The model under review builds one solid part; all positions refer to its coordinate system, in mm. A direction names the side the tool comes from. Coordinates: 2 decimals unless noted, no trailing zeros. Order: outer loops, then holes, each group sorted by start corner. A loop starts at its lowest first (then second) coordinate and runs counter-clockwise, first axis right, second up. Notation, with made-up numbers: (-9, 2.25) -> (10, 2.25) arc R18 ccw to (10, 30.25) -> close; hole circle Ø4 at (56.5, -20). An arc over 180 degrees is marked (long way). Use one line per item in the form item = value. Start each with the question number.
(1) Take a section at C-C (y = -6.5). State the section outline as (x, z) points, then the cut area to 3 significant figures.
(2) Wall thickness on line 1 along Y through (x, z) = (-6.75, 0.35); line 2 along Z through (x, y) = (-9.5, 4.5); line 3 along Y through (x, z) = (8, 0.9): over which ranges is each line inside the solid? List them lowest first.
(3) Take a section at A-A (y = 0.25). State the section outline as (x, z) points.
(4) Insertion check: pin 1 Ø0.5 at (x, z) = (7, 0.5) entering from +Y; pin 2 Ø0.7 at (y, z) = (-8, 2) entering from +X; pin 3 Ø1 at (x, z) = (8, 1.5) entering from -Y. Each pin has a flat end and moves straight along its axis. Give the tip position at first contact, or say it passes through.
(5) Mouldability with a two-part tool opening along X and no side actions: class faces 1 (the flat face through (-8, 9.45, 2)), 2 (the flat face through (-5.55, 7, 2)), 3 (the flat face through (-9.45, -7, 2)), 4 (the cylindrical face through (-5.72, -7.48, 1.09)) as +X half, -X half, draft (parallel to the pull), parting line (faces both ways), or undercut.
(6) Take a section at D-D (x = -7.25). State the section outline as (y, z) points.
(7) For faces 5 (the cylindrical face through (-7.527, -5.723, 1.082)), 6 (the flat face through (9.45, -7, 2)), 7 (the flat face through (-5.55, -7, 2)), 8 (the cylindrical face through (7.47, 9.28, 1.09)), list the 3-axis set-ups (+Z, -Z, +X, -X, +Y, -Y) from which the entire face can be reached by the end or side of a thin tool; tool diameter is ignored.
```python
from build123d import *

# Parameters (mm, degrees)
SKETCH_1_W          = 30
SKETCH_1_H          = 30
EXTRUDE_1_DEPTH     = 2
SKETCH_2_W          = 3
SKETCH_2_H          = 3
EXTRUDE_2_DEPTH     = 1
EXTRUDE_START       = 5
EXTRUDE_3_DEPTH     = 5
CUT_EXTRUDE_1_DEPTH = 29.793271784
FILLET_1_R          = 0.1
FILLET_2_R          = 0.2


with BuildPart() as part:
    # 草图1 → 凸台-拉伸1 (new body)
    with BuildSketch(Plane.XY):
        Rectangle(SKETCH_1_W, SKETCH_1_H)
    extrude(amount=-EXTRUDE_1_DEPTH)

    # 草图2 → 凸台-拉伸2 (add)
    with BuildSketch(Plane.XY):
        with Locations((-7.5, -7.5)):
            Rectangle(SKETCH_2_W, SKETCH_2_H)
        with Locations((7.5, -7.5)):
            Rectangle(SKETCH_2_W, SKETCH_2_H)
    extrude_2 = extrude(amount=EXTRUDE_2_DEPTH)

    # 草图3 → 凸台-拉伸3 (add)
    with BuildSketch(Plane.XZ.offset(EXTRUDE_START)):
        with BuildLine():
            Line((-9.45, 2.5), (-5.55, 2.5))
            Line((-5.55, 2.5), (-5.55, 1.555590279))
            ThreePointArc((-5.55, 1.555590279), (-5.719957697, 1.088161527), (-6, 0.677124344))
            Line((-6, 0.677124344), (-9, 0.677124344))
            ThreePointArc((-9, 0.677124344), (-9.280042303, 1.088161527), (-9.45, 1.555590279))
            Line((-9.45, 1.555590279), (-9.45, 2.5))
        make_face()
        with BuildLine():
            Line((9, 0.677124344), (6, 0.677124344))
            ThreePointArc((6, 0.677124344), (5.719957697, 1.088161527), (5.55, 1.555590279))
            Line((5.55, 1.555590279), (5.55, 2.5))
            Line((5.55, 2.5), (9.45, 2.5))
            Line((9.45, 2.5), (9.45, 1.555590279))
            ThreePointArc((9.45, 1.555590279), (9.280042303, 1.088161527), (9, 0.677124344))
        make_face()
    extrude_3 = extrude(amount=EXTRUDE_3_DEPTH)

    # 草图4 → 切除-拉伸1 (cut, through all)
    with BuildSketch(Plane.ZY.offset(9.45)):
        with BuildLine():
            Line((2.5, -5.5530417), (1.528231876, -5.556437591))
            ThreePointArc((1.528231876, -5.556437591), (1.075676747, -5.72640858), (0.677124344, -6))
            Line((0.677124344, -6), (0.677124344, -5))
            Line((0.677124344, -5), (2.5, -5))
            Line((2.5, -5), (2.5, -5.5530417))
        make_face()
        with BuildLine():
            Line((0.677124344, -10), (2.5, -10))
            Line((2.5, -10), (2.5, -9.45))
            Line((2.5, -9.45), (1.555590279, -9.45))
            ThreePointArc((1.555590279, -9.45), (1.088161527, -9.280042303), (0.677124344, -9))
            Line((0.677124344, -9), (0.677124344, -10))
        make_face()
    cut_extrude_1 = extrude(amount=-CUT_EXTRUDE_1_DEPTH, mode=Mode.SUBTRACT)

    # 镜向1: 凸台-拉伸2, 凸台-拉伸3, 切除-拉伸1 across plane
    add(extrude_2.mirror(Plane.ZX))
    add(extrude_3.mirror(Plane.ZX))
    add(cut_extrude_1.mirror(Plane.ZX), mode=Mode.SUBTRACT)

    # 圆角1
    fillet_1_edges = [part.edges().sort_by_distance(p)[0] for p in [
        (-5.55, -7.50152085, 2.5),
        (-9.45, -7.50152085, 2.5),
        (5.55, -7.50152085, 2.5),
        (9.45, -7.50152085, 2.5),
        (7.5, -9.45, 2.5),
        (-7.5, -9.45, 2.5),
        (7.5, 5.5530417, 2.5),
        (-7.5, 5.5530417, 2.5),
        (-5.55, 7.50152085, 2.5),
        (-9.45, 7.50152085, 2.5),
        (9.45, 7.50152085, 2.5),
        (5.55, 7.50152085, 2.5),
        (7.5, 9.45, 2.5),
        (-7.5, 9.45, 2.5),
        (7.5, -5.5530417, 2.5),
        (-7.5, -5.5530417, 2.5),
    ]]
    fillet(fillet_1_edges, radius=FILLET_1_R)

    # 圆角2
    fillet_2_edges = [part.edges().sort_by_distance(p)[0] for p in [
        (15, 0, -2),
        (0, 15, -2),
        (-15, 0, -2),
        (0, 15, 0),
        (15, 0, 0),
        (0, -15, 0),
        (-15, 0, 0),
        (0, -15, -2),
        (-15, 15, -1),
        (15, 15, -1),
        (15, -15, -1),
        (-15, -15, -1),
    ]]
    fillet(fillet_2_edges, radius=FILLET_2_R)


solid = part.part
```
Findings:
q1.outline = (-15, -1.8) arc R0.2 ccw to (-14.8, -2) -> (14.8, -2) arc R0.2 ccw to (15, -1.8) -> (15, -0.2) arc R0.2 ccw to (14.8, 0) -> (9, 0) -> (9, 0.68) arc R2 ccw to (9.45, 1.56) -> (9.45, 2.4) arc R0.1 ccw to (9.35, 2.5) -> (5.65, 2.5) arc R0.1 ccw to (5.55, 2.4) -> (5.55, 1.56) arc R2 ccw to (6, 0.68) -> (6, 0) -> (-6, 0) -> (-6, 0.68) arc R2 ccw to (-5.55, 1.56) -> (-5.55, 2.4) arc R0.1 ccw to (-5.65, 2.5) -> (-9.35, 2.5) arc R0.1 ccw to (-9.45, 2.4) -> (-9.45, 1.56) arc R2 ccw to (-9, 0.68) -> (-9, 0) -> (-14.8, 0) arc R0.2 ccw to (-15, -0.2) -> close
q1.area = 77.6 mm²
q2.line_1 = -9 to -6, 6 to 9
q2.line_2 = -2 to 0
q2.line_3 = -9.17 to -5.83, 5.83 to 9.17
q3.outline = (-15, -1.8) arc R0.2 ccw to (-14.8, -2) -> (14.8, -2) arc R0.2 ccw to (15, -1.8) -> (15, -0.2) arc R0.2 ccw to (14.8, 0) -> (-14.8, 0) arc R0.2 ccw to (-15, -0.2) -> close
q4.pin_1 = 9.06
q4.pin_2 = 9.45
q4.pin_3 = -9.45
q5.face_1 = draft
q5.face_2 = undercut
q5.face_3 = -X half
q5.face_4 = undercut
q6.outline = (-15, -1.8) arc R0.2 ccw to (-14.8, -2) -> (14.8, -2) arc R0.2 ccw to (15, -1.8) -> (15, -0.2) arc R0.2 ccw to (14.8, 0) -> (9, 0) -> (9, 0.68) arc R2 ccw to (9.45, 1.56) -> (9.45, 2.4) arc R0.1 ccw to (9.35, 2.5) -> (5.65, 2.5) arc R0.1 ccw to (5.55, 2.4) -> (5.56, 1.53) arc R2 ccw to (6, 0.68) -> (6, 0) -> (-6, 0) -> (-6, 0.68) arc R2 ccw to (-5.56, 1.53) -> (-5.55, 2.4) arc R0.1 ccw to (-5.65, 2.5) -> (-9.35, 2.5) arc R0.1 ccw to (-9.45, 2.4) -> (-9.45, 1.56) arc R2 ccw to (-9, 0.68) -> (-9, 0) -> (-14.8, 0) arc R0.2 ccw to (-15, -0.2) -> close
q7.face_5 = +X, -X
q7.face_6 = +Z, +X, +Y, -Y
q7.face_7 = +Z, +Y, -Y
q7.face_8 = +X, -X, +Y
